```python
from build123d import *

# Parameters (mm, degrees)
SKETCH1_W                   = 51
SKETCH1_H                   = 38
SKETCH1_W_2                 = 41
SKETCH1_H_2                 = 21
MAIN_BODY_DEPTH             = 10
SKETCH2_W                   = 41
SKETCH2_H                   = 21
SKETCH2_W_2                 = 39
SKETCH2_H_2                 = 19
END_STOP_DEPTH              = 5
CONTOURING_R                = 1
SKETCH4_W                   = 21
SKETCH4_H                   = 5.5
CLEARANCE_MIDDLE_DEPTH      = 21
EDGE_CONTOURING_R           = 3
INNER_CONTOURING_R          = 2.5
FIT_CONTOURING_R            = 1
SKETCH5_W                   = 15.358498738
SKETCH5_H                   = 54.278463244
SINGLE_CUT_DEPTH            = 52
SKETCH6_W                   = 13
SKETCH6_H                   = 7
CLEARANCE_WIRE_DEPTH        = 6
SKETCH7_W                   = 3
SKETCH7_H                   = 13
WIRE_CAP_DEPTH              = 6
WIRE_CLEARANCE_CONTOURING_R = 1


with BuildPart() as part:
    # Sketch1 → Main Body (new body, symmetric)
    with BuildSketch(Plane(origin=(0, 0, 0), x_dir=(0, 0, -1), z_dir=(1, 0, 0))):
        Rectangle(SKETCH1_W, SKETCH1_H)
        Rectangle(SKETCH1_W_2, SKETCH1_H_2, mode=Mode.SUBTRACT)
    extrude(amount=MAIN_BODY_DEPTH, both=True)

    # Sketch2 → End Stop (add, symmetric)
    with BuildSketch(Plane(origin=(0, 0, 0), x_dir=(0, 0, -1), z_dir=(1, 0, 0))):
        Rectangle(SKETCH2_W, SKETCH2_H)
        Rectangle(SKETCH2_W_2, SKETCH2_H_2, mode=Mode.SUBTRACT)
    extrude(amount=END_STOP_DEPTH, both=True)

    # Contouring
    contouring_edges = [part.edges().sort_by_distance(p)[0] for p in [
        (7.5, 10.5, 20.5),
        (7.5, -10.5, 20.5),
        (7.5, -10.5, -20.5),
        (7.5, 10.5, -20.5),
        (-7.5, 10.5, -20.5),
        (-7.5, 10.5, 20.5),
        (-7.5, -10.5, -20.5),
        (-7.5, -10.5, 20.5),
        (0, 9.5, 19.5),
        (0, -9.5, 19.5),
        (0, 9.5, -19.5),
    ]]
    fillet(contouring_edges, radius=CONTOURING_R)

    # Sketch4 → Clearance - Middle (cut, through all)
    with BuildSketch(Plane(origin=(10, 0, 0), x_dir=(0, 0, -1), z_dir=(1, 0, 0))):
        with Locations((0, 16.25)):
            Rectangle(SKETCH4_W, SKETCH4_H)
        with Locations((0, -16.25)):
            Rectangle(SKETCH4_W, SKETCH4_H)
    extrude(amount=-CLEARANCE_MIDDLE_DEPTH, mode=Mode.SUBTRACT)

    # Edge Contouring
    edge_contouring_edges = [part.edges().sort_by_distance(p)[0] for p in [
        (0, 19, 25.5),
        (0, 19, -25.5),
        (0, -19, -25.5),
        (0, -19, 25.5),
    ]]
    fillet(edge_contouring_edges, radius=EDGE_CONTOURING_R)

    # Inner Contouring
    inner_contouring_edges = [part.edges().sort_by_distance(p)[0] for p in [
        (0, 13.5, 10.5),
        (0, 19, 10.5),
        (0, 19, -10.5),
        (0, 13.5, -10.5),
        (0, -19, -10.5),
        (0, -19, 10.5),
        (0, -13.5, 10.5),
        (0, -13.5, -10.5),
    ]]
    fillet(inner_contouring_edges, radius=INNER_CONTOURING_R)

    # Fit Contouring
    fit_contouring_edges = [part.edges().sort_by_distance(p)[0] for p in [
        (-10, -10.5, 0),
        (-10, 0, -20.5),
        (-10, 0, 20.5),
        (10, 0, -20.5),
        (10, 10.5, 0),
        (-10, 10.5, 0),
        (10, 0, 20.5),
        (10, -10.5, 0),
        (-10, -10.207106781, -20.207106781),
        (-10, -10.207106781, 20.207106781),
        (10, 10.207106781, -20.207106781),
        (-10, 10.207106781, -20.207106781),
        (-10, 10.207106781, 20.207106781),
        (10, 10.207106781, 20.207106781),
        (10, -10.207106781, 20.207106781),
        (10, -10.207106781, -20.207106781),
    ]]
    fillet(fit_contouring_edges, radius=FIT_CONTOURING_R)

    # Sketch5 → Single Cut (cut, through all)
    with BuildSketch(Plane(origin=(0, 0, -25.5), x_dir=(-1, 0, 0), z_dir=(0, 0, -1))):
        with Locations((-11.679249369, 0)):
            Rectangle(SKETCH5_W, SKETCH5_H)
    extrude(amount=-SINGLE_CUT_DEPTH, mode=Mode.SUBTRACT)

    # Sketch6 → Clearance - Wire (cut)
    with BuildSketch(Plane(origin=(0, 0, -25.5), x_dir=(-1, 0, 0), z_dir=(0, 0, -1))):
        Rectangle(SKETCH6_W, SKETCH6_H)
    extrude(amount=-CLEARANCE_WIRE_DEPTH, mode=Mode.SUBTRACT)

    # Sketch7 → Wire Cap (add)
    with BuildSketch(Plane(origin=(0, 0, -25.5), x_dir=(-1, 0, 0), z_dir=(0, 0, -1))):
        with Locations((-5.5, 0)):
            Rectangle(SKETCH7_W, SKETCH7_H)
    extrude(amount=-WIRE_CAP_DEPTH)

    # Wire Clearance Contouring
    wire_clearance_contouring_edges = [part.edges().sort_by_distance(p)[0] for p in [
        (4, -3.5, -22.5),
        (4, 3.5, -22.5),
        (-6.5, -3.5, -23),
        (-6.5, 3.5, -23),
        (4, 6.5, -22.5),
        (7, 6.5, -22.5),
        (7, -6.5, -22.5),
        (4, -6.5, -22.5),
    ]]
    fillet(wire_clearance_contouring_edges, radius=WIRE_CLEARANCE_CONTOURING_R)


solid = part.part
```
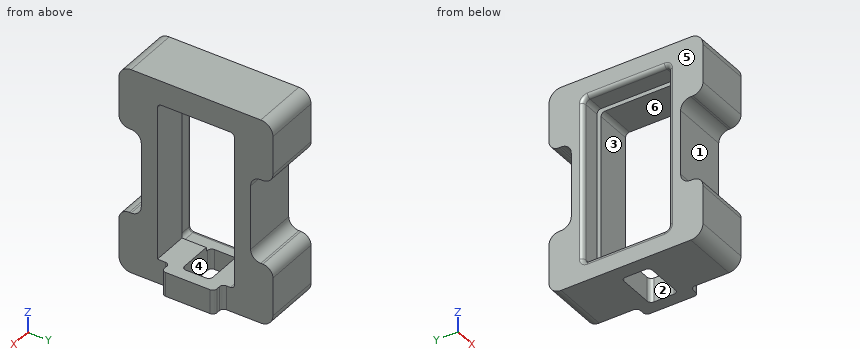
Read the model definition and answer for the solid it produces. Units are mm, in the model's axes. Face numbers are marked on the shaded views. A direction names the side the tool comes from. Coordinates: 2 decimals unless noted, no trailing zeros. Order: outer loops, then holes, each group sorted by start corner. A loop starts at its lowest first (then second) coordinate and runs counter-clockwise, first axis right, second up. Notation, with made-up numbers: (54.25, 51.5) - (91.25, 51.5) arc R18 ccw to (91.25, 80.5) - close; hole circle Ø10 at (10, 11). An arc over 180 degrees is marked (long way). Answer as a JSON object with one key per item and string values. Group by question number.
Item 1: Section B-B (y = -14.5) is taken. Give the vertices of the cut face in (x, z).
Item 2: Consider probe 1 along Z at (x, y) = (-7, -4); probe 2 along Z at (x, y) = (-4, -6); probe 3 along Y at (x, z) = (-4, 5.5). Determine where each line is inside the solid, lowest interval first. Write a range as from..to.
Item 3: A tool of negligible diameter and unlimited length cuts with its end or side. For the marked faces 1, 2 and 3, from which of +Z, -Z, +X, -X, +Y, -Y can it reach the whole face along a straight path? Write none if from no direction.
Item 4: Section C-C (z = 14) is taken. Give the vertices of the cut face in (x, y), plus the area to 3 significant figures.
Item 5: Section A-A (z = -3) is taken. Give the vertices of the cut face in (x, y), plus the area to 3 significant figures.
Item 6: The mould has two halves that part along X. Classify the marked faces 4, 5 and 6: +X half, -X half, draft (parallel to the pull), parting line (faces both ways), or undercut.
Item 7: Flat-ended cylindrical pins translate along their axes: P1, Ø1.5, axis at y = 12.5, z = 4, coming from the +X side; P2, Ø10, axis at x = 0.5, z = 7, coming from the +Y side; P3, Ø2.5, axis at x = -2, z = -6.5, coming from the -Y side; P4, Ø5, axis at y = -5.5, z = -15.5, coming from the -X side. Find the tip coordinate at first contact, or state that the pin passes through.
Results are:
{
 "1": {"outline": "(-10, -25.5) - (4, -25.5) - (4, -10) - (-10, -10) - close; (-10, 10) - (4, 10) - (4, 25.5) - (-10, 25.5) - close"},
 "2": {"probe 1": "z = -25.5..-20.5, 20.5..25.5", "probe 2": "z = -25.5..-19.5, 19.5..25.5", "probe 3": "y = -13.5..-9.5, 9.5..13.5"},
 "3": {"face 1": "+X, -X, -Y", "face 2": "-Z", "face 3": "+X, -X"},
 "4": {"outline": "(-10, -19) - (4, -19) - (4, -9.5) - (-5, -9.5) - (-5, -10.5) - (-9, -10.5) arc R1 ccw to (-10, -11.5) - close; (-10, 11.5) arc R1 ccw to (-9, 10.5) - (-5, 10.5) - (-5, 9.5) - (4, 9.5) - (4, 19) - (-10, 19) - close", "area": "256 mm^2"},
 "5": {"outline": "(-10, -13.5) - (4, -13.5) - (4, -9.5) - (-5, -9.5) - (-5, -10.5) - (-9, -10.5) arc R1 ccw to (-10, -11.5) - close; (-10, 11.5) arc R1 ccw to (-9, 10.5) - (-5, 10.5) - (-5, 9.5) - (4, 9.5) - (4, 13.5) - (-10, 13.5) - close", "area": "102 mm^2"},
 "6": {"face 4": "undercut", "face 5": "-X half", "face 6": "draft"},
 "7": {"P1": "stops at x = 4", "P2": "stops at y = 18.79", "P3": "stops at y = -13.5", "P4": "passes through"}
}
